from build123d import *

# Parameters (mm, degrees)
BOSS_EXTRUDE1_DEPTH = 20
FILLET1_R           = 1


with BuildPart() as part:
    # Sketch1 → Boss-Extrude1 (new body)
    with BuildSketch(Plane.XY):
        with BuildLine():
            Line((5.679190751, 0), (19, 0))
            ThreePointArc((19, 0), (19.707106781, 0.292893219), (20, 1))
            Line((20, 1), (20, 2))
            ThreePointArc((20, 2), (19.707106781, 2.707106781), (19, 3))
            Line((19, 3), (5, 3))
            ThreePointArc((5, 3), (3.585786438, 3.585786438), (3, 5))
            Line((3, 5), (3, 19))
            ThreePointArc((3, 19), (2.707106781, 19.707106781), (2, 20))
            Line((2, 20), (1, 20))
            ThreePointArc((1, 20), (0.292893219, 19.707106781), (0, 19))
            Line((0, 19), (0, 2))
            ThreePointArc((0, 2), (0.585786438, 0.585786438), (2, 0))
            Line((2, 0), (5.679190751, 0))
        make_face()
    extrude(amount=BOSS_EXTRUDE1_DEPTH)

    # Fillet1
    fillet1_edges = [part.edges().sort_by_distance(p)[0] for p in [
        (2.707106781, 19.707106781, 20),
        (12, 3, 0),
        (19.707106781, 2.707106781, 0),
        (20, 1.5, 0),
        (19.707106781, 0.292893219, 0),
        (10.5, 0, 0),
        (0.585786438, 0.585786438, 0),
        (0, 10.5, 0),
        (0.292893219, 19.707106781, 0),
        (1.5, 20, 0),
        (1.5, 20, 20),
        (2.707106781, 19.707106781, 0),
        (3, 12, 0),
        (3.585786438, 3.585786438, 0),
        (0.292893219, 19.707106781, 20),
        (0, 10.5, 20),
        (0.585786438, 0.585786438, 20),
        (10.5, 0, 20),
        (19.707106781, 0.292893219, 20),
        (20, 1.5, 20),
        (19.707106781, 2.707106781, 20),
        (3.585786438, 3.585786438, 20),
        (12, 3, 20),
        (3, 12, 20),
    ]]
    fillet(fillet1_edges, radius=FILLET1_R)


solid = part.part
Geometry: final body of the model. Coordinates: model frame, mm. A direction names the side the tool comes from. Coordinates: 2 decimals unless noted, no trailing zeros. Order: outer loops, then holes, each group sorted by start corner. A loop starts at its lowest first (then second) coordinate and runs counter-clockwise, first axis right, second up. Notation, with made-up numbers: M -3.75,64 L 16.25,64 A20 cw 16.25,99 Z; hole C -24,40.25 d11. An arc over 180 degrees is marked long. One line per question, with ' | ' between items. Start each with the question number.
Item 1: Ray query, probe 1 along X at (y, z) = (12.25, 14); probe 2 along X at (y, z) = (2.75, 5.5). Return the intervals inside material, ascending. Write a range as [from, to].
Item 2: Draft query along Z for faces 6 (the cylindrical face through (19.715, 2.699, 9.874)), 7 (the cylindrical face through (19.715, 1.507, 0.301)), 8 (the cylindrical face through (11.902, 2.715, 19.699)). Return one class per face: released by +Z, released by -Z, zero draft, split by the parting line, or undercut.
Item 3: Cut plane C-C, the plane z = 7. Return the cut outline in (x, y), then the cut area to 3 significant figures.
Item 4: Pin query (flat end, axial travel): pin 1 Ø5 at (y, z) = (14.5, 15) entering from +X; pin 2 Ø2 at (x, z) = (13, 18) entering from +Y. Return the tip coordinate at first contact, or that it passes through.
Item 5: Set-up query: faces 1 (the cylindrical face through (11.902, 2.715, 0.301)), 2 (the cylindrical face through (0.285, 10.381, 19.699)), 3 (the flat face through (3, 12, 10)), 4 (the cylindrical face through (2.715, 12.098, 19.699)), 5 (the cylindrical face through (0.301, 19.715, 9.874)). Return all of +Z, -Z, +X, -X, +Y, -Y with unobstructed straight access to the full face (end or side cutting, diameter ignored); none if empty.
Item 6: Cut plane A-A, the plane y = 15.5. Return the cut outline in (x, z), then the cut area to 3 significant figures.
A:
1) probe 1: x = [0, 3] | probe 2: x = [0, 19.66]
2) face 6: zero draft | face 7: released by -Z | face 8: released by +Z
3) outline: M 0,2 A2 ccw 2,0 L 19,0 A1 ccw 20,1 L 20,2 A1 ccw 19,3 L 5,3 A2 cw 3,5 L 3,19 A1 ccw 2,20 L 1,20 A1 ccw 0,19 Z | area: 110 mm2
4) pin 1: stops at x = 3 | pin 2: stops at y = 3
5) face 1: -Z, +X, +Y | face 2: +Z, -X, +Y, -Y | face 3: +Z, -Z, +X, +Y | face 4: +Z, +X, +Y | face 5: +Z, -Z, -X, +Y
6) outline: M 0,1 A1 ccw 1,0 L 2,0 A1 ccw 3,1 L 3,19 A1 ccw 2,20 L 1,20 A1 ccw 0,19 Z | area: 59.1 mm2
